```python
from build123d import *

# Parameters (mm, degrees)
SKETCH1_R           = 3.5
BOSS_EXTRUDE2_DEPTH = 55
SKETCH7_W           = 68.999652055
SKETCH7_H           = 50.415620377
CUT_EXTRUDE5_DEPTH  = 13
SKETCH19_W          = 74.859412742
SKETCH19_H          = 60.725118028
CUT_EXTRUDE7_DEPTH  = 13
CUT_EXTRUDE9_DEPTH  = 55


with BuildPart() as part:
    # Sketch1 → Boss-Extrude2 (new body)
    with BuildSketch(Plane(origin=(0, 0, 0), x_dir=(1, 0, 0), z_dir=(0, 1, 0))):
        with BuildLine():
            Line((-77.297393365, -66.943127962), (112.637979465, -57.343127962))
            add(Edge.make_bspline(
                [(112.637979465, -57.343127962), (125.082628436, -56.027724614), (133.287763268, -44.662014668), (142.702606635, -37.943127962)],
                knots=[0, 0, 0, 0, 1, 1, 1, 1], degree=3))
            Line((142.702606635, -37.943127962), (146.202606635, -37.943127962))
            Line((146.202606635, -37.943127962), (146.302606635, -37.943127962))
            ThreePointArc((146.302606635, -37.943127962), (150.120983253, -36.36150458), (151.702606635, -32.543127962))
            Line((151.702606635, -32.543127962), (151.702606635, 23.656872038))
            ThreePointArc((151.702606635, 23.656872038), (150.120983253, 27.475248656), (146.302606635, 29.056872038))
            Line((146.302606635, 29.056872038), (146.202606635, 29.056872038))
            Line((146.202606635, 29.056872038), (142.702606635, 29.056872038))
            add(Edge.make_bspline(
                [(112.637979465, 48.456872038), (125.082628436, 47.14146869), (133.287763268, 35.775758744), (142.702606635, 29.056872038)],
                knots=[0, 0, 0, 0, 1, 1, 1, 1], degree=3))
            Line((112.637979465, 48.456872038), (-77.297393365, 58.056872038))
            add(Edge.make_bspline(
                [(-77.297393365, 58.056872038), (-97.47829568, 56.558543187), (-92.669908534, 31.299380259), (-112.297393365, 29.056872038)],
                knots=[0, 0, 0, 0, 1, 1, 1, 1], degree=3))
            Line((-112.297393365, 29.056872038), (-115.797393365, 29.056872038))
            Line((-115.797393365, 29.056872038), (-115.897393365, 29.056872038))
            ThreePointArc((-115.897393365, 29.056872038), (-119.715769983, 27.475248656), (-121.297393365, 23.656872038))
            Line((-121.297393365, 23.656872038), (-121.297393365, -32.543127962))
            ThreePointArc((-121.297393365, -32.543127962), (-119.715769983, -36.36150458), (-115.897393365, -37.943127962))
            Line((-115.897393365, -37.943127962), (-115.797393365, -37.943127962))
            Line((-115.797393365, -37.943127962), (-112.297393365, -37.943127962))
            add(Edge.make_bspline(
                [(-77.297393365, -66.943127962), (-97.47829568, -65.444799111), (-92.669908534, -40.185636183), (-112.297393365, -37.943127962)],
                knots=[0, 0, 0, 0, 1, 1, 1, 1], degree=3))
        make_face()
        with Locations((-112.297393365, 20.556872038)):
            Circle(SKETCH1_R, mode=Mode.SUBTRACT)
        with Locations((-112.297393365, -29.443127962)):
            Circle(SKETCH1_R, mode=Mode.SUBTRACT)
        with Locations((142.702606635, -29.443127962)):
            Circle(SKETCH1_R, mode=Mode.SUBTRACT)
        with Locations((142.702606635, 20.556872038)):
            Circle(SKETCH1_R, mode=Mode.SUBTRACT)
    extrude(amount=-BOSS_EXTRUDE2_DEPTH)

    # Sketch7 → Cut-Extrude5 (cut)
    with BuildSketch(Plane.ZY.offset(121.297393365)):
        with Locations((4.333112833, -30.707810189)):
            Rectangle(SKETCH7_W, SKETCH7_H)
    extrude(amount=-CUT_EXTRUDE5_DEPTH, mode=Mode.SUBTRACT)

    # Sketch19 → Cut-Extrude7 (cut)
    with BuildSketch(Plane(origin=(151.702606635, 0, 0), x_dir=(0, 0, -1), z_dir=(1, 0, 0))):
        with Locations((-5.097493458, -35.862559014)):
            Rectangle(SKETCH19_W, SKETCH19_H)
    extrude(amount=-CUT_EXTRUDE7_DEPTH, mode=Mode.SUBTRACT)

    # Sketch24 → Cut-Extrude9 (cut)
    with BuildSketch(Plane(origin=(0, 0, 0), x_dir=(1, 0, 0), z_dir=(0, 1, 0))):
        with BuildLine():
            Line((-97.297393365, 31.372357528), (-97.297393365, -40.258643174))
            add(Edge.make_bspline(
                [(-97.297393365, -40.258643174), (-97.055392699, -40.522543308), (-96.818465561, -40.791519395), (-95.29604309, -42.586141239), (-94.180102109, -44.221795649), (-92.114981147, -47.600331907), (-91.167558943, -49.344344007), (-89.714260063, -51.939679671), (-89.224013692, -52.801383116), (-88.197386212, -54.493312492), (-87.661405753, -55.323638026), (-86.787164869, -56.520642624), (-86.483908233, -56.911472942), (-85.845311529, -57.670997258), (-85.510678135, -58.038515471), (-84.461423347, -59.080983609), (-83.697062972, -59.699960103), (-82.417122679, -60.472101656), (-81.975749173, -60.698816325), (-81.073807536, -61.09027214), (-80.611895531, -61.255932259), (-79.196960523, -61.672670039), (-78.210701758, -61.84358461), (-77.219838786, -61.93282554)],
                knots=[0.352672192, 0.352672192, 0.352672192, 0.352672192, 0.375, 0.375, 0.5, 0.5, 0.625, 0.625, 0.6875, 0.6875, 0.75, 0.75, 0.78125, 0.78125, 0.8125, 0.8125, 0.875, 0.875, 0.90625, 0.90625, 0.9375, 0.9375, 1, 1, 1, 1], degree=3))
            Line((-77.219838786, -61.93282554), (112.240105599, -52.356855361))
            add(Edge.make_bspline(
                [(112.240105599, -52.356855361), (113.717382254, -52.189730891), (115.132971643, -51.8376863), (117.182437857, -51.088035578), (117.853343768, -50.801431656), (119.174145437, -50.165241611), (119.826422425, -49.814165646), (121.732436005, -48.696872923), (122.940710016, -47.866553193), (125.285242411, -46.107289747), (126.421126606, -45.177833586), (127.59402171, -44.178301992), (127.648334729, -44.131926563), (127.702606635, -44.085499704)],
                knots=[0, 0, 0, 0, 0.125, 0.125, 0.1875, 0.1875, 0.25, 0.25, 0.375, 0.375, 0.5, 0.5, 0.506074438, 0.506074438, 0.506074438, 0.506074438], degree=3))
            Line((127.702606635, -44.085499704), (127.702606635, 35.199241787))
            add(Edge.make_bspline(
                [(127.702606635, 35.199241787), (127.656893723, 35.238347374), (126.494699106, 36.231003566), (125.312312668, 37.199657877), (123.548827323, 38.524500877), (122.950515573, 38.954402998), (121.735559113, 39.776761834), (121.118108697, 40.169868377), (119.227839741, 41.28046867), (117.917675896, 41.930280463), (115.836701988, 42.695260765), (115.130607863, 42.912098814), (113.700996756, 43.257880714), (112.975983658, 43.387349472), (112.240105599, 43.470599437)],
                knots=[0.494878569, 0.494878569, 0.494878569, 0.494878569, 0.5, 0.625, 0.625, 0.6875, 0.6875, 0.75, 0.75, 0.875, 0.875, 0.9375, 0.9375, 1, 1, 1, 1], degree=3))
            Line((112.240105599, 43.470599437), (-77.219838786, 53.046569616))
            add(Edge.make_bspline(
                [(-77.219838786, 53.046569616), (-78.226254375, 52.955927957), (-79.213157443, 52.784359124), (-80.65236022, 52.356330798), (-81.126202061, 52.184487982), (-82.053330615, 51.775193987), (-82.497083796, 51.5419399), (-83.346280845, 51.020113337), (-83.751740407, 50.731563524), (-84.52795848, 50.104355813), (-84.899500865, 49.764992502), (-85.964937473, 48.68741183), (-86.589708432, 47.913990928), (-87.747790314, 46.308292885), (-88.280321037, 45.475513671), (-89.301365793, 43.781629681), (-89.789527485, 42.920298168), (-91.239394158, 40.326896414), (-92.188900691, 38.584245442), (-94.255960588, 35.221000735), (-95.371079537, 33.60184943), (-96.859865551, 31.858322069), (-97.076237995, 31.613508704), (-97.297393365, 31.372357528)],
                knots=[0, 0, 0, 0, 0.0625, 0.0625, 0.09375, 0.09375, 0.125, 0.125, 0.15625, 0.15625, 0.1875, 0.1875, 0.25, 0.25, 0.3125, 0.3125, 0.375, 0.375, 0.5, 0.5, 0.625, 0.625, 0.645748558, 0.645748558, 0.645748558, 0.645748558], degree=3))
        make_face()
    extrude(amount=-CUT_EXTRUDE9_DEPTH, mode=Mode.SUBTRACT)


solid = part.part
```
Geometry check sheet. Reference: the model listing, model coordinates, mm. A direction names the side the tool comes from. Coordinates: 2 decimals unless noted, no trailing zeros. Write each loop counter-clockwise with the first axis right and the second up, starting at its lowest first coordinate (ties: lowest second). Pieces come first, ordered by that corner, then holes. Notation, with made-up numbers: M 55,2 L 78,2 A18 cw 78,21 Z; hole C 50,83 d9. An arc over 180 degrees is marked long. Answer as a JSON object with one key per item and string values.
1. Tool access check on faces 1 (the cylindrical face through (-119.67, -2.71, -27.52)), 2 (the flat face through (18.84, -27.12, -48.19)), 3 (the flat face through (-108.297, -30, 4)). Record the directions out of +Z, -Z, +X, -X, +Y, -Y that give a thin tool (end or side, any length) a straight path to the whole face; none if there is none.
Answers below:
{"face 1": "-Z, -X, +Y, -Y", "face 2": "+Y, -Y", "face 3": "+Z, -Z, -X, -Y"}
2. Section check A-A, the plane z = -6. Enter the section's corners in (x, y).
Answers below:
{"outline": "M -121.3,-5.5 L -108.3,-5.5 L -108.3,-55 L -97.3,-55 L -97.3,0 L -121.3,0 Z; M 127.7,-55 L 138.7,-55 L 138.7,-5.5 L 151.7,-5.5 L 151.7,0 L 127.7,0 Z"}
3. Section check B-B, the plane x = 27. Enter the section's corners in (y, z), plus the area to 3 significant figures.
Answers below:
{"outline": "M -55,-52.79 L 0,-52.79 L 0,-47.78 L -55,-47.78 Z; M -55,56.67 L 0,56.67 L 0,61.67 L -55,61.67 Z", "area": "551 mm²"}
4. Scan lines: L1, parallel to X at y = -24, z = -11.5; L2, parallel to X at y = -4, z = -18.5; L3, parallel to Z at x = 10, y = -25. Record each from-to range of solid material in increasing order.
Answers below:
{"L1": "x = -108.3 to -97.3, 127.7 to 138.7", "L2": "x = -121.3 to -115.13, -109.47 to -97.3, 127.7 to 139.87, 145.53 to 151.7", "L3": "z = -53.64 to -48.64, 57.52 to 62.53"}
5. Draft check along X on faces 4 (the flat face through (138.703, -30, 5)), 5 (the flat face through (127.703, -27, 5)), 6 (the flat face through (15, -55, 60)), 7 (the cylindrical face through (-109.064, -2.712, -19.216)). Enter one of: released by +X, released by -X, zero draft, split by the parting line, or undercut.
Answers below:
{"face 4": "released by +X", "face 5": "undercut", "face 6": "zero draft", "face 7": "undercut"}
6. Go/stop test with flat-tipped pins: pin 1 Ø16.5 at (y, z) = (-40.5, -12) entering from +X; pin 2 Ø1.5 at (x, y) = (-74.5, -38.5) entering from +Z; pin 3 Ø1.1 at (x, y) = (144, -3.5) entering from -Z; pin 4 Ø6.5 at (x, z) = (-112.3, 29.44) entering from +Y. Record where each tip stops, or that it passes through.
Answers below:
{"pin 1": "stops at x = 138.7", "pin 2": "stops at z = 66.84", "pin 3": "stops at z = -29.06", "pin 4": "passes through"}
